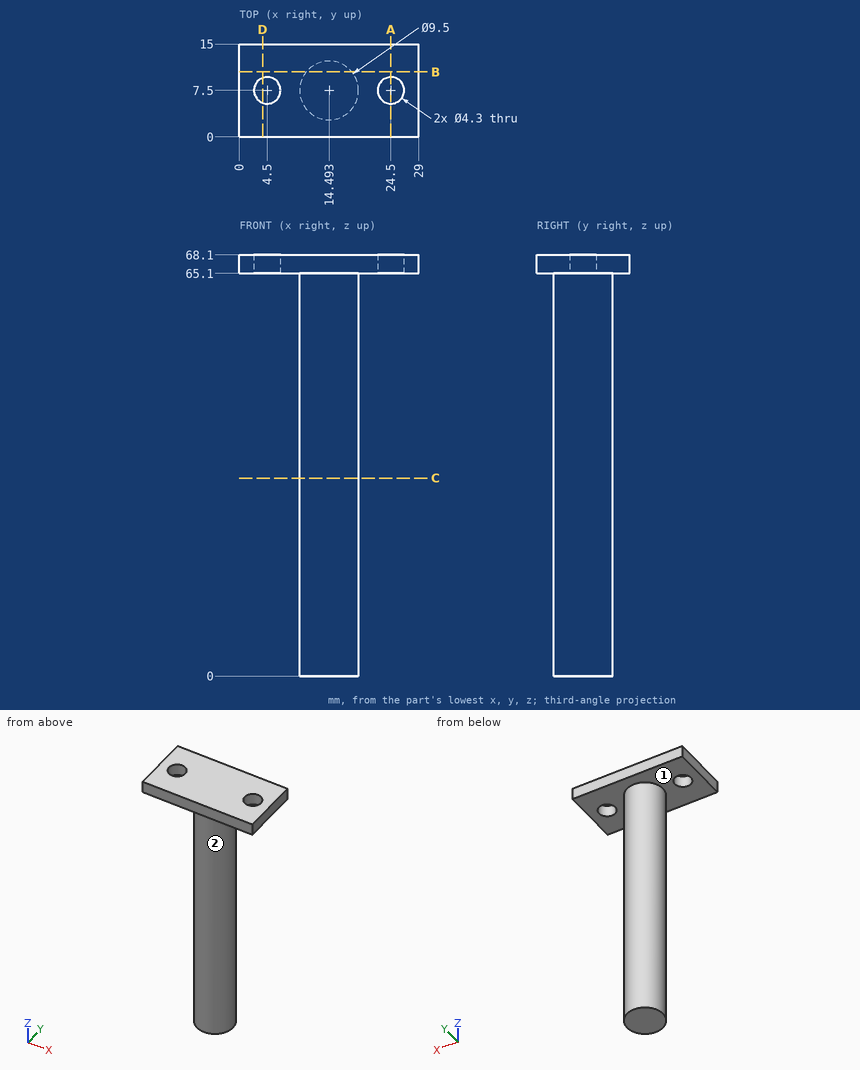
Study the drawing (mm; zero at the part's minimum x, y, z) and answer. Coordinates: 2 decimals unless noted, no trailing zeros. Loops run counter-clockwise (first coordinate to the right, second up) from the corner with the lowest first, then second, coordinate; pieces in that order, holes last. Notation, with made-up numbers: (18, 37.5) -> (29, 37.5) arc R19 cw to (29, 65.5) -> close; hole circle Ø3 at (67, -36). An arc over 180 degrees is marked (long way). Answer in a Markdown table with one row per item. Add a question column.
1. The part is cut by section A-A, the plane x = 24.5. Write down the section's boundary in (y, z).
2. Consider line 1 (Z direction, x = 10.75, y = 12.75); line 2 (Y direction, x = 4.5, z = 67.15); line 3 (Y direction, x = 12.5, z = 53.5). Determine where each line is inside the solid, lowest interval first. Write a range as [from, to].
3. The part is cut by section C-C, the plane z = 32. Write down the section's boundary in (x, y), then the cut area to 3 significant figures.
4. The part is cut by section B-B, the plane y = 10.5. Write down the section's boundary in (x, z) (1 decimal).
5. The part is cut by section D-D, the plane x = 3.75. Write down the section's boundary in (y, z) (1 decimal), then the cut area to 3 significant figures.
6. Flat-ended cylindrical pins translate along their axes: P1, Ø1, axis at x = 17, z = 24, coming from the -Y side (1 decimal); P2, Ø2, axis at y = 10, z = 50.5, coming from the +X side; P3, Ø4, axis at y = 8, z = 24.5, coming from the -X side; P4, Ø4, axis at x = 7, z = 59, coming from the -Y side. Find the tip coordinate at first contact, or state that the pin passes through.
7. Determine the mould class of the marked faces 1 and 2 for opening direction X: +X half, -X half, draft (parallel to the pull), parting line (faces both ways), or undercut.
Answer below:
| question | item | result |
|---|---|---|
| 1 | outline | (0, 65.1) -> (5.35, 65.1) -> (5.35, 68.1) -> (0, 68.1) -> close; (9.65, 65.1) -> (15, 65.1) -> (15, 68.1) -> (9.65, 68.1) -> close |
| 2 | line 1 | [65.1, 68.1] |
| 2 | line 2 | [0, 5.35], [9.65, 15] |
| 2 | line 3 | [3.19, 11.81] |
| 3 | outline | circle Ø9.5 at (14.49, 7.5) |
| 3 | area | 70.9 mm2 |
| 4 | outline | (0, 65.1) -> (10.8, 65.1) -> (10.8, 0) -> (18.2, 0) -> (18.2, 65.1) -> (29, 65.1) -> (29, 68.1) -> (0, 68.1) -> close |
| 5 | outline | (0, 65.1) -> (5.5, 65.1) -> (5.5, 68.1) -> (0, 68.1) -> close; (9.5, 65.1) -> (15, 65.1) -> (15, 68.1) -> (9.5, 68.1) -> close |
| 5 | area | 32.9 mm2 |
| 6 | P1 | y = 3.2 |
| 6 | P2 | x = 19 |
| 6 | P3 | x = 9.74 |
| 6 | P4 | through |
| 7 | face 1 | draft |
| 7 | face 2 | parting line |
